Could you check a few things on this drawing? It's one solid part, dimensions in mm from its lowest x, y, z. A direction names the side the tool comes from. Give positions to 0.01 mm unless a question says otherwise; leave off trailing zeros. Order: outer loops, then holes, each group sorted by start corner. A loop starts at its lowest first (then second) coordinate and runs counter-clockwise, first axis right, second up.
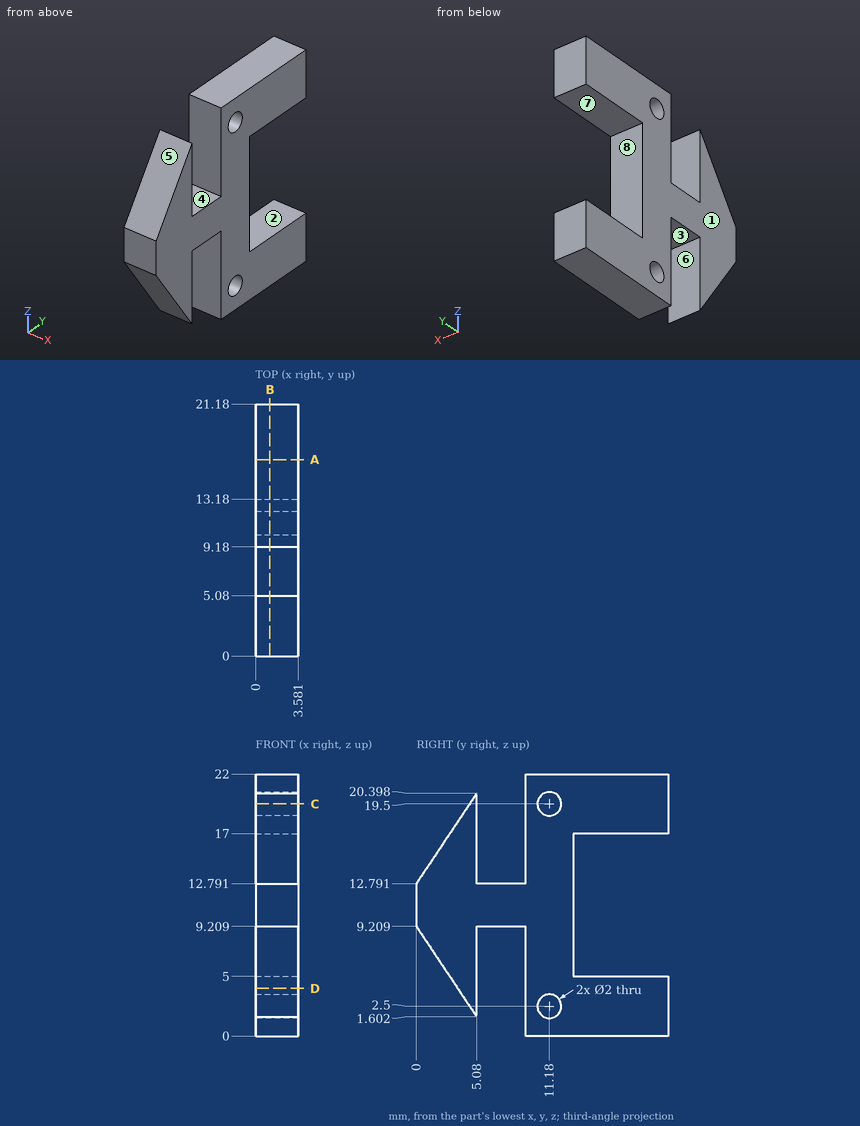
1) We'd pull the mould along Y, two halves only. Please class the marked faces 5, 6, 7 and 8: +Y half, -Y half, draft (parallel to the pull), parting line (faces both ways), or undercut.
2) Suppose I cut it at A-A (y = 16.5). Please give me the cut outline in (x, z).
3) I'm going to push flat-ended pins straight in: pin 1 Ø2 at (x, z) = (1.5, 14.5) entering from +Y; pin 2 Ø10 at (y, z) = (15, 6.5) entering from +X; pin 3 Ø1.5 at (x, z) = (2, 4) entering from -Y; pin 4 Ø1.2 at (y, z) = (11.18, 2.5) entering from -X. Where does each tip first touch, or does it pass through?
4) If I drill on line 1 (Y direction, x = 2.3, z = 19.5); line 2 (Z direction, x = 2.75, y = 11.5); line 3 (Z direction, x = 0.45, y = 14.25), over which ranges is the centre line in solid material (lowest first)?
5) Suppose I cut it at D-D (z = 4). Please give me the cut outline in (x, y).
6) Suppose I cut it at B-B (x = 1.2). Please give me the cut outline in (y, z).
7) Suppose I cut it at C-C (z = 19.5). Please give me the cut outline in (x, y).
8) Which directions (+Z, -Z, +X, -X, +Y, -Y) give clear straight access to the entire face, cutting with the end or side of a thin tool? Please do the marked faces 1, 2, 3 and 4.
Results:
1. face 5: -Y half
1. face 6: undercut
1. face 7: draft
1. face 8: +Y half
2. outline: (0, 0) - (3.58, 0) - (3.58, 5) - (0, 5) - close; (0, 17) - (3.58, 17) - (3.58, 22) - (0, 22) - close
3. pin 1: stops at y = 13.18
3. pin 2: stops at x = 3.58
3. pin 3: stops at y = 2.98
3. pin 4: passes through
4. line 1: y = 4.48 to 5.08, 9.18 to 10.18, 12.18 to 21.18
4. line 2: z = 0 to 1.55, 3.45 to 18.55, 20.45 to 22
4. line 3: z = 0 to 5, 17 to 22
5. outline: (0, 3.48) - (3.58, 3.48) - (3.58, 5.08) - (0, 5.08) - close; (0, 9.18) - (3.58, 9.18) - (3.58, 21.18) - (0, 21.18) - close
6. outline: (0, 9.21) - (5.08, 1.6) - (5.08, 9.21) - (9.18, 9.21) - (9.18, 0) - (21.18, 0) - (21.18, 5) - (13.18, 5) - (13.18, 17) - (21.18, 17) - (21.18, 22) - (9.18, 22) - (9.18, 12.79) - (5.08, 12.79) - (5.08, 20.4) - (0, 12.79) - close; hole circle Ø2 at (11.18, 2.5); hole circle Ø2 at (11.18, 19.5)
7. outline: (0, 4.48) - (3.58, 4.48) - (3.58, 5.08) - (0, 5.08) - close; (0, 9.18) - (3.58, 9.18) - (3.58, 10.18) - (0, 10.18) - close; (0, 12.18) - (3.58, 12.18) - (3.58, 21.18) - (0, 21.18) - close
8. face 1: +Z, -Z, -X, +Y, -Y
8. face 2: +X, -X, +Y
8. face 3: -Z, +X, -X
8. face 4: +Z, +X, -X
